from build123d import *

# Parameters (mm, degrees)
SKETCH3_R             = 5.1
SKETCH3_R_2           = 3.1
BOSS_EXTRUDE2_DEPTH   = 4
BOSS_EXTRUDE2_2_DEPTH = 4
CUT_EXTRUDE1_DEPTH    = 4
BOSS_EXTRUDE3_START   = -23.25
BOSS_EXTRUDE3_DEPTH   = 46.5
SKETCH7_W             = 9.658407056
SKETCH7_H             = 6.6
CUT_EXTRUDE2_DEPTH    = 2
FILLET1_R             = 8
FILLET2_R             = 6
FILLET3_R             = 10
FILLET4_R             = 15


with BuildPart() as part:
    # Sketch3 → Boss-Extrude2 (new body)
    with BuildSketch(Plane.XY):
        with Locations((-116.546102611, -10.445456474)):
            Circle(SKETCH3_R)
        with Locations((-116.546102611, -10.445456474)):
            Circle(SKETCH3_R_2, mode=Mode.SUBTRACT)
    extrude(amount=BOSS_EXTRUDE2_DEPTH)


with BuildPart() as body_2:
    # Sketch3 → Boss-Extrude2 2 (new body)
    with BuildSketch(Plane.XY):
        with Locations(Location((-26.546102611, -10.445456474, 0), (0, 0, 180))):
            Circle(SKETCH3_R)
        with Locations(Location((-26.546102611, -10.445456474, 0), (0, 0, 180))):
            Circle(SKETCH3_R_2, mode=Mode.SUBTRACT)
    extrude(amount=BOSS_EXTRUDE2_2_DEPTH)


with BuildPart() as cut_extrude1_tool:
    # Sketch4 → Cut-Extrude1 (new body)
    with BuildSketch(Plane.XY.offset(4)):
        Polygon((-116.546102611, -10.445456474), (-134.15945469, -20.614530038), (-98.932750532, -20.614530038), align=None)
        Polygon((-26.546102611, -10.445456474), (-8.932750532, -20.614530038), (-44.15945469, -20.614530038), align=None)
    extrude(amount=-CUT_EXTRUDE1_DEPTH)


with BuildPart() as part_1:
    add(part.part)

    # Cut-Extrude1: cut by cut_extrude1_tool
    add(cut_extrude1_tool.part, mode=Mode.SUBTRACT)


with BuildPart() as body_2_1:
    add(body_2.part)

    # Cut-Extrude1: cut by cut_extrude1_tool
    add(cut_extrude1_tool.part, mode=Mode.SUBTRACT)


with BuildPart() as body_3:
    # Mirror2: mirrored copy
    add(part_1.part.mirror(Plane.XY.offset(23.25)))


with BuildPart() as body_4:
    # Mirror2 2: mirrored copy
    add(body_2_1.part.mirror(Plane.XY.offset(23.25)))


with BuildPart() as part_2:
    add(part_1.part)

    add(body_2_1.part)  # Boss-Extrude3 merges body 2

    add(body_3.part)  # Boss-Extrude3 merges body 3

    add(body_4.part)  # Boss-Extrude3 merges body 4
    # Sketch6 → Boss-Extrude3 (add)
    with BuildSketch(Plane.XY.offset(23.25).offset(BOSS_EXTRUDE3_START)):
        with BuildLine():
            Line((-121.546102611, -7.345456474), (-106.100588572, -7.345456474))
            ThreePointArc((-106.100588572, -7.345456474), (-71.546102611, 7.404543526), (-36.99161665, -7.345456474))
            Line((-36.99161665, -7.345456474), (-21.546102611, -7.345456474))
            Line((-21.546102611, -7.345456474), (-21.546102611, -5.345456474))
            Line((-21.546102611, -5.345456474), (-36.148186006, -5.345456474))
            ThreePointArc((-36.148186006, -5.345456474), (-71.546102611, 9.404543526), (-106.944019216, -5.345456474))
            Line((-106.944019216, -5.345456474), (-121.546102611, -5.345456474))
            Line((-121.546102611, -5.345456474), (-121.546102611, -7.345456474))
        make_face()
    extrude(amount=BOSS_EXTRUDE3_DEPTH)

    # Sketch7 → Cut-Extrude2 (cut)
    with BuildSketch(Plane(origin=(0, -5.345456474, 0), x_dir=(1, 0, 0), z_dir=(0, 1, 0))):
        with Locations((-118.016899083, -12)):
            Rectangle(SKETCH7_W, SKETCH7_H)
        with Locations((-118.016899083, -34.5)):
            Rectangle(SKETCH7_W, SKETCH7_H)
        with Locations((-25.075306139, -34.5)):
            Rectangle(SKETCH7_W, SKETCH7_H)
        with Locations((-25.075306139, -12)):
            Rectangle(SKETCH7_W, SKETCH7_H)
    extrude(amount=-CUT_EXTRUDE2_DEPTH, mode=Mode.SUBTRACT)

    # Fillet1
    fillet1_edges = [part_2.edges().sort_by_distance(p)[0] for p in [
        (-36.148186006, -5.345456474, 23.25),
        (-106.944019216, -5.345456474, 23.25),
    ]]
    fillet(fillet1_edges, radius=FILLET1_R)

    # Fillet2
    fillet2_edges = [part_2.edges().sort_by_distance(p)[0] for p in [
        (-106.100588572, -7.345456474, 23.25),
        (-36.99161665, -7.345456474, 23.25),
    ]]
    fillet(fillet2_edges, radius=FILLET2_R)

    # Fillet3
    # the kernel refuses this fillet: 10 mm, written as the material it adds along each edge
    with BuildSketch(Plane(origin=(-112.496411265, -7.345456474, 4), x_dir=(0.9974995155199412, 0.07067330852226088, 0), z_dir=(0, 0, -1)), Plane(origin=(-30.595793957, -7.345456474, 42.5), x_dir=(-0.9974995155199468, 0.07067330852218129, 0), z_dir=(0, 0, 1))) as fillet3_piece_1:
        with BuildLine():
            CenterArc((9.270136929, 9.512895054), FILLET3_R, 206.369759274, 45.673490189)
            Line((0.310673789, 5.07127145), (-0.585272525, 4.62710909))
            ThreePointArc((-0.585272525, 4.62710909), (-0.16632442, 2.555341186), (-0.835029885, 0.550204591))
            Line((-0.835029885, 0.550204591), (0.070673309, -0.997499516))
            ThreePointArc((0.070673309, -0.997499516), (3.983986296, -0.720239455), (5.878847867, -0.951289505))
            Line((5.878847867, -0.951289505), (6.187146873, 0))
        make_face()
    extrude(amount=4)
    with BuildSketch(Plane(origin=(-112.496411265, -7.345456474, 42.5), x_dir=(0.9974995155199412, 0.07067330852226088, 0), z_dir=(0, 0, 1)), Plane(origin=(-30.595793957, -7.345456474, 4), x_dir=(-0.9974995155199468, 0.07067330852218129, 0), z_dir=(0, 0, -1))) as fillet3_piece_2:
        with BuildLine():
            CenterArc((9.270136929, -9.512895054), FILLET3_R, 107.956750537, 45.673490189)
            Line((0.310673789, -5.07127145), (-0.585272525, -4.62710909))
            ThreePointArc((-0.585272525, -4.62710909), (-0.16632442, -2.555341186), (-0.835029885, -0.550204591))
            Line((-0.835029885, -0.550204591), (0.070673309, 0.997499516))
            ThreePointArc((0.070673309, 0.997499516), (3.983986296, 0.720239455), (5.878847867, 0.951289505))
            Line((5.878847867, 0.951289505), (6.187146873, 0))
        make_face()
    extrude(amount=4)

    # Fillet4
    # the kernel refuses this fillet: 15 mm, written as the material it adds along each edge
    with BuildSketch(Plane(origin=(-120.595793957, -7.345456474, 4), x_dir=(-0.37317563120438824, -0.9277607171438153, 0), z_dir=(0, 0, -1)), Plane(origin=(-22.496411265, -7.345456474, 42.5), x_dir=(0.3731756312044104, -0.9277607171438064, 0), z_dir=(0, 0, 1))) as fillet4_piece_1:
        with BuildLine():
            CenterArc((6.743777429, 14.452908836), FILLET4_R, 244.789631476, 9.688258422)
            Line((0.354632032, 0.881659038), (0, 0))
            ThreePointArc((0, 0), (1.364812099, 0.186010996), (2.729624198, 0))
        make_face()
    extrude(amount=4)
    with BuildSketch(Plane(origin=(-120.595793957, -7.345456474, 42.5), x_dir=(-0.37317563120438824, -0.9277607171438153, 0), z_dir=(0, 0, 1))) as fillet4_piece_2:
        with BuildLine():
            CenterArc((6.743777429, -14.452908836), FILLET4_R, 105.522110102, 9.688258422)
            Line((0.354632032, -0.881659038), (0, 0))
            ThreePointArc((0, 0), (1.364812099, -0.186010996), (2.729624198, 0))
        make_face()
    extrude(amount=4)
    with BuildSketch(Plane(origin=(-22.496411265, -7.345456474, 4), x_dir=(1, 0, 0), z_dir=(0, 0, -1))) as fillet4_piece_3:
        with BuildLine():
            CenterArc((15.925454466, 0.863138406), FILLET4_R, 173.610509594, 9.688258422)
            ThreePointArc((1.018629233, 2.532438103), (0.681888311, 1.196804281), (0, 0))
            Line((0, 0), (0.950308654, 0))
        make_face()
    extrude(amount=4)


solid = part_2.part
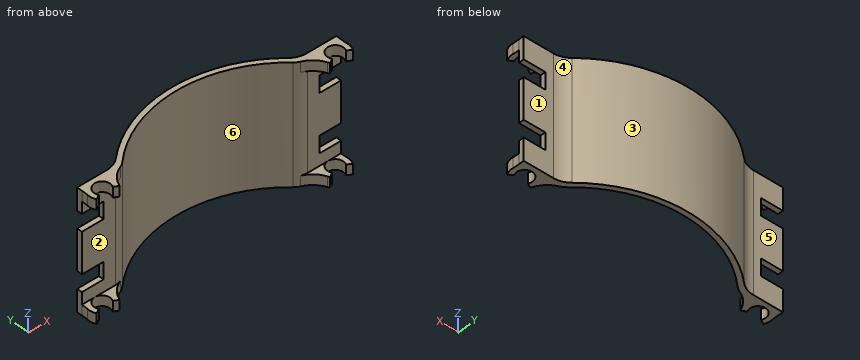
Model file for the job. Use its own axes, mm. Face numbers are marked on the shaded views. A direction names the side the tool comes from. Give positions to 0.01 mm unless a question says otherwise; leave off trailing zeros. Loops run counter-clockwise (first coordinate to the right, second up) from the corner with the lowest first, then second, coordinate; pieces in that order, holes last.
1) Saw through at D-D (x = -87.5). Write the cut outline in (y, z), plus the area to 3 significant figures.
2) Flat gauge pins, fed straight in: pin 1 Ø1 at (y, z) = (-6.5, 21.5) entering from -X; pin 2 Ø10 at (y, z) = (-1.5, 5.5) entering from +X; pin 3 Ø6 at (x, z) = (-84, 9) entering from +Y; pin 4 Ø6 at (x, y) = (-76.5, 1.5) entering from +Z. Where does each tip first touch, or does it go through?
3) Saw through at B-B (y = 2.5). Write the cut outline in (x, z).
4) Tool access for the marked faces 1, 2 and 3: list every direction of +Z, -Z, +X, -X, +Y, -Y with a clear straight run to the whole face (end or side of a thin tool).
5) Pull direction X, two halves, no side cores. Call the marked faces 4, 5 and 6: +X half, -X half, draft (parallel to the pull), parting line (faces both ways), or undercut.
6) Saw through at A-A (z = 19.5). Write the cut outline in (x, y), plus the area to 3 significant figures.
7) Wall check: line 1 (X direction, y = 1.5, z = 27); line 2 (X direction, y = 2.5, z = 22); line 3 (Y direction, x = -47, z = 22). Give the ranges that are in metal, low to high.
8) Saw through at C-C (z = 35.5). Write the cut outline in (x, y), plus the area to 3 significant figures.
Answer block:
1. outline: (4.67, 0) - (6.78, 0) - (6.78, 46.5) - (4.67, 46.5) - close
1. area: 98.4 mm2
2. pin 1: stops at x = -121.55
2. pin 2: stops at x = -21.55
2. pin 3: stops at y = 8.5
2. pin 4: passes through
3. outline: (-96.86, 0) - (-92.65, 0) - (-92.65, 46.5) - (-96.86, 46.5) - close; (-50.44, 0) - (-46.23, 0) - (-46.23, 46.5) - (-50.44, 46.5) - close
4. face 1: +Z, -Z, +X, +Y
4. face 2: +X, -X, -Y
4. face 3: +Z, -Z, +Y
5. face 4: +X half
5. face 5: draft
5. face 6: undercut
6. outline: (-121.55, -7.35) - (-108.57, -7.35) arc R6 ccw to (-104.45, -5.7) arc R47.85 cw to (-38.64, -5.7) arc R6 ccw to (-34.52, -7.35) - (-21.55, -7.35) - (-21.55, -5.35) - (-32.96, -5.35) arc R8 cw to (-38.29, -3.31) arc R49.85 ccw to (-104.8, -3.31) arc R8 cw to (-110.13, -5.35) - (-121.55, -5.35) - close
6. area: 217 mm2
7. line 1: x = -98.48 to -94.57, -48.52 to -44.61
7. line 2: x = -96.86 to -92.65, -50.44 to -46.23
7. line 3: y = 0.63 to 2.94
8. outline: (-113.19, -7.35) - (-108.57, -7.35) arc R6 ccw to (-104.45, -5.7) arc R47.85 cw to (-38.64, -5.7) arc R6 ccw to (-34.52, -7.35) - (-29.9, -7.35) - (-29.9, -5.35) - (-32.96, -5.35) arc R8 cw to (-38.29, -3.31) arc R49.85 ccw to (-104.8, -3.31) arc R8 cw to (-110.13, -5.35) - (-113.19, -5.35) - close
8. area: 184 mm2
